```python
from build123d import *

# Parameters (mm, degrees)
F0_W     = 127
F0_H     = 127
F1_DEPTH = 127
F2_W     = 76.2
F2_H     = 63.5
F3_DEPTH = 76.2
F4_R     = 25.4
F5_DEPTH = 76.2
F6_W     = 38.1
F6_H     = 63.5
F7_DEPTH = 50.8
F8_R     = 38.1
F9_SIZE  = 25.4


with BuildPart() as f1:
    # F0 (on Front) → F1 (new body)
    with BuildSketch(Plane.XZ):
        with Locations((0.941295, 0.866529)):
            Rectangle(F0_W, F0_H)
    extrude(amount=F1_DEPTH)

    # F2 (on face) → F3 (cut)
    with BuildSketch(Plane.XY.offset(64.366529)):
        with Locations((26.341295, -95.25)):
            Rectangle(F2_W, F2_H)
    extrude(amount=-F3_DEPTH, mode=Mode.SUBTRACT)

    # F4 (on face) → F5 (cut)
    with BuildSketch(Plane.XY.offset(-11.833471)):
        with Locations((24.607655, -93.949772)):
            Circle(F4_R)
    extrude(amount=-F5_DEPTH, mode=Mode.SUBTRACT)

    # F6 (on face) → F7 (cut)
    with BuildSketch(Plane.XY.offset(64.366529)):
        with Locations((7.291295, -31.75)):
            Rectangle(F6_W, F6_H)
    extrude(amount=-F7_DEPTH, mode=Mode.SUBTRACT)

    # F8
    f8_edges = [f1.edges().sort_by_distance(p)[0] for p in [
        (-37.158705, -127, 64.366529),
    ]]
    fillet(f8_edges, radius=F8_R)

    # F9
    f9_edges = [f1.edges().sort_by_distance(p)[0] for p in [
        (64.441295, -31.75, 64.366529),
    ]]
    chamfer(f9_edges, length=F9_SIZE)


solid = f1.part
```
CAD build for the part. Positions are in the model's coordinates, mm. A direction names the side the tool comes from. Coordinates: 2 decimals unless noted, no trailing zeros. Write each loop counter-clockwise with the first axis right and the second up, starting at its lowest first coordinate (ties: lowest second). Pieces come first, ordered by that corner, then holes.
(1) Cut at A-A, the plane z = 15.5. List the corners of the cut face in (x, y), and give its area (3 significant figures).
(2) 3-axis set-ups, long thin cutter, end or side, ignore diameter. For faces 4 (the face through (26.341, -32, 39)), 5 (the face through (51, -95, -11.833)), 6 (the face through (-11.759, -64, 27)): which of +Z, -Z, +X, -X, +Y, -Y reach the whole face in a straight line?
(3) Cut at D-D, the plane y = -26.5. List the corners of the cut face in (x, z).
(4) Cut at B-B, the plane y = -114. List the corners of the cut face in (x, z), and give its area (3 significant figures).
(5) Cut at C-C, the plane x = 41.5. List the corners of the cut face in (y, z), and give its area (3 significant figures).
(6) Drill centre lines: probe 1 along X at (y, z) = (-41.5, 17.5); probe 2 along X at (y, z) = (-95, -42.5); probe 3 along Z at (x, y) = (1.5, -76.5). Where is each one in solid material? Low to high.
(7) Two-plate mould, pull along Y, no slides. Class faces 1 (the face through (-36.803, -116.135, 52.909)), 2 (the face through (7, -31, 13.567)), 3 (the face through (4.451, -109.405, -36.878)): +Y half, -Y half, draft (parallel to the pull), parting line (faces both ways), or undercut.
Geometry says:
1. outline: (-62.56, -127) - (-11.76, -127) - (-11.76, 0) - (-62.56, 0) - close; (26.34, -63.5) - (64.44, -63.5) - (64.44, 0) - (26.34, 0) - close
1. area: 8,870 mm2
2. face 4: +Z, +Y, -Y
2. face 5: +Z, +X, -Y
2. face 6: +Z, -Y
3. outline: (-62.56, -62.63) - (64.44, -62.63) - (64.44, 38.97) - (39.04, 64.37) - (26.34, 64.37) - (26.34, 13.57) - (-11.76, 13.57) - (-11.76, 64.37) - (-62.56, 64.37) - close
4. outline: (-62.56, -62.63) - (9.01, -62.63) - (9.01, -11.83) - (-11.76, -11.83) - (-11.76, 54.93) - (-62.56, 54.93) - close; (40.2, -62.63) - (64.44, -62.63) - (64.44, -11.83) - (40.2, -11.83) - close
4. area: 8,260 mm2
5. outline: (-127, -62.63) - (-112.92, -62.63) - (-112.92, -11.83) - (-127, -11.83) - close; (-74.98, -62.63) - (0, -62.63) - (0, 61.91) - (-63.5, 61.91) - (-63.5, -11.83) - (-74.98, -11.83) - close
5. area: 9,210 mm2
6. probe 1: x = -62.56 to -11.76, 26.34 to 64.44
6. probe 2: x = -62.56 to -0.77, 49.99 to 64.44
6. probe 3: z = -62.63 to -11.83
7. face 1: -Y half
7. face 2: draft
7. face 3: undercut
